Autodesk Inventor part; units mm, degrees
ref_plane "YZ Plane" through (0, 0, 0) normal (1, 0, 0) x (0, 1, 0)
ref_plane "XZ Plane" through (0, 0, 0) normal (0, 1, 0) x (-1, 0, 0)
ref_plane "XY Plane" through (0, 0, 0) normal (0, 0, 1) x (1, 0, 0)
sketch "Sketch1" plane through (0, 0, 0) normal (0, 0, 1) x (1, 0, 0)
  line L0 (3.6662, 6.35) -> (7.3323, 0)
  line L1 (7.3323, 0) -> (3.6662, -6.35)
  line L2 (3.6662, -6.35) -> (-3.6662, -6.35)
  line L3 (-3.6662, -6.35) -> (-7.3323, 0)
  line L4 (-7.3323, 0) -> (-3.6662, 6.35)
  line L5 (-3.6662, 6.35) -> (3.6662, 6.35)
  circle A0 centre (0, 0) radius 12.7
  circle A1 centre (0, 0) radius 7.3323 construction
  dimension "d0" = 12.7
  dimension "d2" = 25.4
  dimension "d3" = 5.3677
extrude "Extrusion1" add sketch "Sketch1" against normal blind 19.05
sketch "Sketch2" plane through (0, 0, -19.05) normal (0, 0, -1) x (-1, 0, 0)
  line L0 (7.3323, 0) -> (3.6662, -6.35)
  line L1 (3.6662, -6.35) -> (-3.6662, -6.35)
  line L2 (-3.6662, -6.35) -> (-7.3323, 0)
  line L3 (-7.3323, 0) -> (-3.6662, 6.35)
  line L4 (-3.6662, 6.35) -> (3.6662, 6.35)
  line L5 (3.6662, 6.35) -> (7.3323, 0)
  line L6 (7.3323, 0) -> (3.6662, -6.35)
  line L7 (-10.9985, 19.05) -> (10.9985, 19.05)
  line L8 (10.9985, 19.05) -> (21.997, 0)
  line L9 (21.997, 0) -> (10.9985, -19.05)
  line L10 (10.9985, -19.05) -> (-10.9985, -19.05)
  line L11 (-10.9985, -19.05) -> (-21.997, 0)
  line L12 (-21.997, 0) -> (-10.9985, 19.05)
  point P0 (0, 0)
  point P1 (0, 0)
  point P2 (0, 0)
  dimension "d7" = 12.7
  dimension "d10" = 38.1
extrude "Extrusion3" add sketch "Sketch2" along normal blind 6.35
thicken "Thicken Internal Hex Hold" operation add thickness 0.1905 both sides no extend neighbours yes toward (0, 1, 0) faces at (1.2221, 6.35, -16.9333) (-4.8882, 4.2333, -16.9333) (1.2221, 14.8167, -25.4) (6.1103, -2.1167, -16.9333) (1.2221, -6.35, -16.9333) (-4.8882, -4.2333, -16.9333)
thicken "Reduce Size of Bushing Fitting" operation add thickness 0.1905 both sides no extend neighbours yes toward (-0.9870503, 0.1604113, 0) faces at (12.5355, -2.0372, -12.7)
equation "\"d13\" = printSpacing"
equation "\"d14\" = printSpacing"
equation "\"d15\" = printSpacing"
equation "\"d16\" = printSpacing"
equation "\"hexSize\" = 12.7"
equation "\"printSpacing\" = 0.1905"
properties part number "1_2x1-hexBushing" material "PC/ABS Plastic"
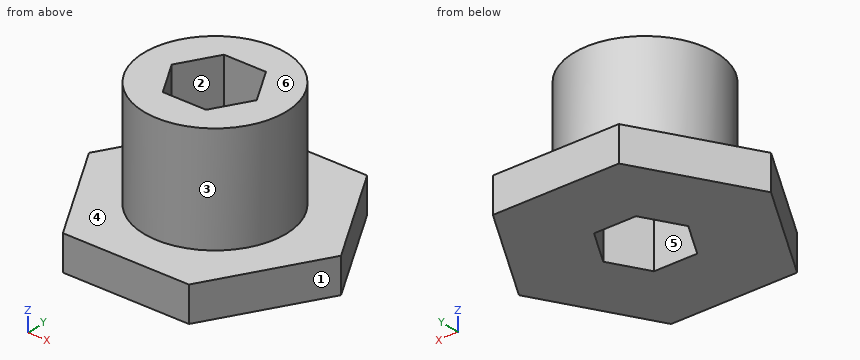
Could you check a few things on this model? Use its own coordinates, in mm. Face numbers are marked on the shaded views. A direction names the side the tool comes from. Give positions to 0.01 mm unless a question says otherwise; leave off trailing zeros. Order: outer loops, then holes, each group sorted by start corner. A loop starts at its lowest first (then second) coordinate and runs counter-clockwise, first axis right, second up. Notation, with made-up numbers: (27.5, 7.25) -> (70.5, 7.25) arc R16 ccw to (70.5, 12.25) -> close; hole circle Ø11 at (-9, 31). An arc over 180 degrees is marked (long way). Answer in a Markdown table with one row per item. Add a question column.
Item 1: For the marked faces 5 and 6, which set-ups out of +Z, -Z, +X, -X, +Y, -Y let a thin tool reach every point of the face, with its end or its side?
Item 2: Imagine slicing it at B-B (z = -3.25). List the corners of the cut face in (x, y) for me, and give its area (3 significant figures).
Item 3: Please list where these lines run through material, in increasing order: probe 1 along Z at (x, y) = (-10.5, 14.5); probe 2 along Y at (x, z) = (-7, -20.25); probe 3 along X at (y, z) = (0.5, -19).
Item 4: I'm going to push flat-ended pins straight in: P1, Ø3.5, axis at x = -1, z = -12, coming from the -Y side; P2, Ø5, axis at x = 13.5, y = -8, coming from the +Z side; P3, Ø8, axis at x = -11, z = -9.5, coming from the +Y side. Where does each tip first touch, or does it pass through?
Item 5: Imagine slicing it at C-C (y = -9). List the corners of the cut face in (x, z) for me, and give its area (3 significant figures).
Item 6: Imagine slicing it at A-A (x = 0). List the corners of the cut face in (y, z) for me, and give its area (3 significant figures).
Item 7: Imagine slicing it at D-D (x = -5.5). List the corners of the cut face in (y, z) for me.
Item 8: We'd pull the mould along Y, two halves only. Please class the marked faces 1, 2, 3 and 4: pulls with the +Y half, pulls with the -Y half, needs draft (parallel to the pull), parting line crosses it, or undercut.
Result:
| question | item | result |
|---|---|---|
| 1 | face 5 | +Z, -Z |
| 1 | face 6 | +Z, +X, -X, +Y, -Y |
| 2 | outline | circle Ø25.02 at (0, 0); hole (-7.55, 0) -> (-3.78, -6.54) -> (3.78, -6.54) -> (7.44, -0.19) -> (3.56, 6.54) -> (-3.78, 6.54) -> close |
| 2 | area | 345 mm2 |
| 3 | probe 1 | -25.21 to -19.05 |
| 3 | probe 2 | -19.05 to -0.96, 0.96 to 19.05 |
| 3 | probe 3 | -12.5 to -7.26, 7.04 to 12.5 |
| 4 | P1 | y = -12.51 |
| 4 | P2 | z = -19.05 |
| 4 | P3 | y = 10.37 |
| 5 | outline | (-16.8, -25.21) -> (16.8, -25.21) -> (16.8, -19.05) -> (8.69, -19.05) -> (8.69, 0) -> (-8.69, 0) -> (-8.69, -19.05) -> (-16.8, -19.05) -> close |
| 5 | area | 538 mm2 |
| 6 | outline | (-19.05, -25.21) -> (-6.54, -25.21) -> (-6.54, 0) -> (-12.51, 0) -> (-12.51, -19.05) -> (-19.05, -19.05) -> close; (6.54, -25.21) -> (19.05, -25.21) -> (19.05, -19.05) -> (12.51, -19.05) -> (12.51, 0) -> (6.54, 0) -> close |
| 6 | area | 382 mm2 |
| 7 | outline | (-19.05, -25.21) -> (-3.55, -25.21) -> (-3.55, 0) -> (-11.24, 0) -> (-11.24, -19.05) -> (-19.05, -19.05) -> close; (3.55, -25.21) -> (19.05, -25.21) -> (19.05, -19.05) -> (11.24, -19.05) -> (11.24, 0) -> (3.55, 0) -> close |
| 8 | face 1 | pulls with the -Y half |
| 8 | face 2 | undercut |
| 8 | face 3 | parting line crosses it |
| 8 | face 4 | needs draft |
